Here's how the part is built. I have some questions about the finished solid (model axes, mm). Face numbers are marked on the shaded views. Round coordinates to 2 decimals unless told otherwise and drop trailing zeros. Loops run counter-clockwise (first coordinate to the right, second up) from the corner with the lowest first, then second, coordinate; pieces in that order, holes last. Notation, with made-up numbers: M 38.5,72.25 L 94.5,72.25 A15 ccw 94.5,77.25 Z; hole C 83.25,83.25 d7. An arc over 180 degrees is marked long. Use a Markdown table: item, result.
from build123d import *

# Parameters (mm, degrees)
SKETCH1_W                     = 262.636
SKETCH1_H                     = 3.175
BASE_FLANGE1_DEPTH            = 80.5688
CUT_EXTRUDE1_DEPTH            = 155.096817886
EDGE_FLANGE2_DEPTH            = 148.4376
EDGE_FLANGE3_DEPTH            = 249.936
EDGE_FLANGE4_DEPTH            = 148.4376
EDGE_FLANGE5_DEPTH            = 249.936
CSK_FOR_M5_SFHCS1_D           = 5.3
CSK_FOR_M5_SFHCS1_CSINK_D     = 11.2
CSK_FOR_M5_SFHCS1_CSINK_ANGLE = 90
CUT_EXTRUDE3_REACH            = 165.583
SKETCH18_W                    = 102.743
SKETCH18_H                    = 52.92295
FILLET2_R                     = 9.525
FILLET3_R                     = 6.35
FILLET4_R                     = 3.175


# Sheet-metal steps are written as plain solids
with BuildPart() as part:
    # Sketch1 → Base-Flange1 (new, symmetric)
    with BuildSketch(Plane.XY):
        with Locations((0, -1.5875)):
            Rectangle(SKETCH1_W, SKETCH1_H)
    extrude(amount=BASE_FLANGE1_DEPTH, both=True)

    # Sketch2 → Cut-Extrude1 (cut, through all)
    with BuildSketch(Plane(origin=(0, 0, 0), x_dir=(-1, 0, 0), z_dir=(0, 1, 0))):
        Polygon((131.318, -80.5688), (131.318, -74.2188), (124.968, -80.5688), align=None)
        Polygon((131.318, 74.2188), (124.968, 80.5688), (131.318, 80.5688), align=None)
        Polygon((-131.318, 80.5688), (-124.968, 80.5688), (-131.318, 74.2188), align=None)
        Polygon((-124.968, -80.5688), (-131.318, -80.5688), (-131.318, -74.2188), align=None)
    extrude(amount=-CUT_EXTRUDE1_DEPTH, mode=Mode.SUBTRACT)

    # Edge-Flange2 section (across the edge) → Edge-Flange2 (add)
    with BuildSketch(Plane(origin=(134.493, 0, 74.2188), x_dir=(-1, 0, 0), z_dir=(0, 0, -1))):
        with BuildLine():
            Line((-3.175, 3.175), (-3.175, 15.875))
            Line((-3.175, 15.875), (0, 15.875))
            Line((0, 15.875), (0, 3.175))
            ThreePointArc((0, 3.175), (0.92993597, 0.92993597), (3.175, 0))
            Line((3.175, 0), (3.175, -3.175))
            ThreePointArc((3.175, -3.175), (-1.315128061, -1.315128061), (-3.175, 3.175))
        make_face()
    extrude(amount=EDGE_FLANGE2_DEPTH)

    # Edge-Flange3 section (across the edge) → Edge-Flange3 (add)
    with BuildSketch(Plane(origin=(-124.968, 0, 83.7438), x_dir=(0, 0, -1), z_dir=(1, 0, 0))):
        with BuildLine():
            Line((-3.175, 3.175), (-3.175, 15.875))
            Line((-3.175, 15.875), (0, 15.875))
            Line((0, 15.875), (0, 3.175))
            ThreePointArc((0, 3.175), (0.92993597, 0.92993597), (3.175, 0))
            Line((3.175, 0), (3.175, -3.175))
            ThreePointArc((3.175, -3.175), (-1.315128061, -1.315128061), (-3.175, 3.175))
        make_face()
    extrude(amount=EDGE_FLANGE3_DEPTH)

    # Edge-Flange4 section (across the edge) → Edge-Flange4 (add)
    with BuildSketch(Plane(origin=(-134.493, 0, -74.2188), x_dir=(1, 0, 0), z_dir=(0, 0, 1))):
        with BuildLine():
            Line((-3.175, 3.175), (-3.175, 15.875))
            Line((-3.175, 15.875), (0, 15.875))
            Line((0, 15.875), (0, 3.175))
            ThreePointArc((0, 3.175), (0.92993597, 0.92993597), (3.175, 0))
            Line((3.175, 0), (3.175, -3.175))
            ThreePointArc((3.175, -3.175), (-1.315128061, -1.315128061), (-3.175, 3.175))
        make_face()
    extrude(amount=EDGE_FLANGE4_DEPTH)

    # Edge-Flange5 section (across the edge) → Edge-Flange5 (add)
    with BuildSketch(Plane(origin=(124.968, 0, -83.7438), x_dir=(0, 0, 1), z_dir=(-1, 0, 0))):
        with BuildLine():
            Line((-3.175, 3.175), (-3.175, 15.875))
            Line((-3.175, 15.875), (0, 15.875))
            Line((0, 15.875), (0, 3.175))
            ThreePointArc((0, 3.175), (0.92993597, 0.92993597), (3.175, 0))
            Line((3.175, 0), (3.175, -3.175))
            ThreePointArc((3.175, -3.175), (-1.315128061, -1.315128061), (-3.175, 3.175))
        make_face()
    extrude(amount=EDGE_FLANGE5_DEPTH)

    # CSK for M5 SFHCS1 (through all)
    with Locations(Plane.XZ.offset(3.175)):
        with Locations((-35, -15.75415), (35, -15.75415), (35, 2.24585), (-35, 2.24585)):
            CounterSinkHole(CSK_FOR_M5_SFHCS1_D / 2, CSK_FOR_M5_SFHCS1_CSINK_D / 2, counter_sink_angle=CSK_FOR_M5_SFHCS1_CSINK_ANGLE)

    # Sketch18 → Cut-Extrude3 (cut, up to next)
    with BuildSketch(Plane(origin=(0, 0, 0), x_dir=(1, 0, 0), z_dir=(0, 1, 0)), mode=Mode.PRIVATE) as cut_extrude3_sk1:
        with Locations((-60.8965, -41.407325)):
            Rectangle(SKETCH18_W, SKETCH18_H)
    cut_extrude3_tool1 = extrude(cut_extrude3_sk1.sketch, amount=-CUT_EXTRUDE3_REACH, mode=Mode.PRIVATE) & part.part
    # Sketch18 → Cut-Extrude3 (cut, up to next)
    with BuildSketch(Plane(origin=(0, 0, 0), x_dir=(1, 0, 0), z_dir=(0, 1, 0)), mode=Mode.PRIVATE) as cut_extrude3_sk2:
        with Locations((60.8965, -41.407325)):
            Rectangle(SKETCH18_W, SKETCH18_H)
    cut_extrude3_tool2 = extrude(cut_extrude3_sk2.sketch, amount=-CUT_EXTRUDE3_REACH, mode=Mode.PRIVATE) & part.part
    # Sketch18 → Cut-Extrude3 (cut, up to next)
    with BuildSketch(Plane(origin=(0, 0, 0), x_dir=(1, 0, 0), z_dir=(0, 1, 0)), mode=Mode.PRIVATE) as cut_extrude3_sk3:
        Polygon((-93.218, 28.45415), (-93.218, 10.45415), (-112.268, 10.45415), (-112.268, 65.62295), (-9.525, 65.62295), (-9.525, 28.45415), align=None)
    cut_extrude3_tool3 = extrude(cut_extrude3_sk3.sketch, amount=-CUT_EXTRUDE3_REACH, mode=Mode.PRIVATE) & part.part
    # Sketch18 → Cut-Extrude3 (cut, up to next)
    with BuildSketch(Plane(origin=(0, 0, 0), x_dir=(1, 0, 0), z_dir=(0, 1, 0)), mode=Mode.PRIVATE) as cut_extrude3_sk4:
        Polygon((9.525, 65.62295), (112.268, 65.62295), (112.268, 10.45415), (93.218, 10.45415), (93.218, 28.45415), (9.525, 28.45415), align=None)
    cut_extrude3_tool4 = extrude(cut_extrude3_sk4.sketch, amount=-CUT_EXTRUDE3_REACH, mode=Mode.PRIVATE) & part.part
    add(cut_extrude3_tool1.solids().sort_by_distance((-60.8965, 0, 41.407325))[0], mode=Mode.SUBTRACT)
    add(cut_extrude3_tool2.solids().sort_by_distance((60.8965, 0, 41.407325))[0], mode=Mode.SUBTRACT)
    add(cut_extrude3_tool3.solids().sort_by_distance((-64.344381, 0, -44.765774))[0], mode=Mode.SUBTRACT)
    add(cut_extrude3_tool4.solids().sort_by_distance((64.344381, 0, -44.765774))[0], mode=Mode.SUBTRACT)

    # Fillet2
    fillet2_edges = [part.edges().sort_by_distance(p)[0] for p in [
        (112.268, -1.5875, 14.94585),
        (112.268, -1.5875, 67.8688),
        (9.525, -1.5875, 67.8688),
        (9.525, -1.5875, 14.94585),
        (-112.268, -1.5875, -65.62295),
        (-9.525, -1.5875, -65.62295),
        (-9.525, -1.5875, -28.45415),
        (-93.218, -1.5875, -28.45415),
        (9.525, -1.5875, -28.45415),
        (9.525, -1.5875, -65.62295),
        (112.268, -1.5875, -65.62295),
        (93.218, -1.5875, -28.45415),
        (-9.525, -1.5875, 14.94585),
        (-9.525, -1.5875, 67.8688),
        (-112.268, -1.5875, 67.8688),
        (-112.268, -1.5875, 14.94585),
    ]]
    fillet(fillet2_edges, radius=FILLET2_R)

    # Fillet3
    fillet3_edges = [part.edges().sort_by_distance(p)[0] for p in [
        (-112.268, -1.5875, -10.45415),
        (-93.218, -1.5875, -10.45415),
        (112.268, -1.5875, -10.45415),
        (93.218, -1.5875, -10.45415),
    ]]
    fillet(fillet3_edges, radius=FILLET3_R)

    # Fillet4
    fillet4_edges = [part.edges().sort_by_distance(p)[0] for p in [
        (-136.0805, 15.875, -74.2188),
        (-136.0805, 15.875, 74.2188),
        (124.968, 15.875, -85.3313),
        (-124.968, 15.875, -85.3313),
        (136.0805, 15.875, 74.2188),
        (136.0805, 15.875, -74.2188),
        (-124.968, 15.875, 85.3313),
        (124.968, 15.875, 85.3313),
    ]]
    fillet(fillet4_edges, radius=FILLET4_R)


solid = part.part
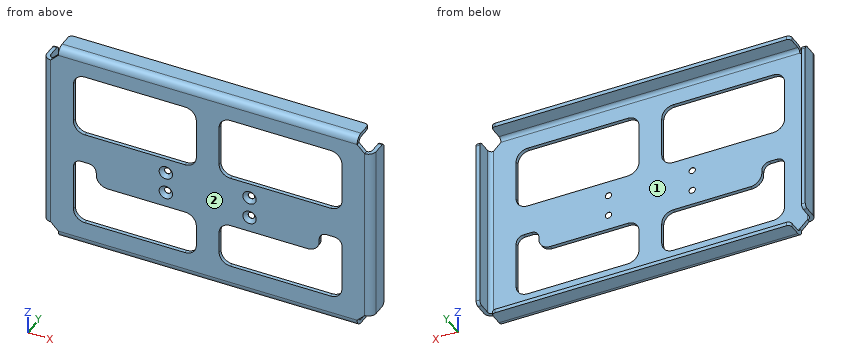
1. Imagine slicing it at B-B, the plane z = -43. Write out the boundary of the cut face in (x, y) (3 decimals), then the cut area to 3 significant figures.
Answer sheet:
| item | result |
|---|---|
| outline | M -137.668,3.175 A6.35 ccw -131.318,-3.175 L -112.268,-3.175 L -112.268,0 L -131.318,0 A3.175 cw -134.493,3.175 L -134.493,15.875 L -137.668,15.875 Z; M -9.525,-3.175 L 9.525,-3.175 L 9.525,0 L -9.525,0 Z; M 112.268,-3.175 L 131.318,-3.175 A6.35 ccw 137.668,3.175 L 137.668,15.875 L 134.493,15.875 L 134.493,3.175 A3.175 cw 131.318,0 L 112.268,0 Z |
| area | 310 mm2 |
2. We'd pull the mould along X, two halves only. Please class the marked faces 1 and 2: +X half, -X half, draft (parallel to the pull), parting line (faces both ways), or undercut.
Answer sheet:
| item | result |
|---|---|
| face 1 | undercut |
| face 2 | draft |
3. Imagine slicing it at A-A, the plane x = -24. Write out the boundary of the cut face in (y, z) (3 decimals), then the cut area to 3 significant figures.
Answer sheet:
| item | result |
|---|---|
| outline | M -3.175,-80.569 A6.35 ccw 3.175,-86.919 L 15.875,-86.919 L 15.875,-83.744 L 3.175,-83.744 A3.175 cw 0,-80.569 L 0,-65.623 L -3.175,-65.623 Z; M -3.175,-28.454 L 0,-28.454 L 0,14.946 L -3.175,14.946 Z; M -3.175,67.869 L 0,67.869 L 0,80.569 A3.175 cw 3.175,83.744 L 15.875,83.744 L 15.875,86.919 L 3.175,86.919 A6.35 ccw -3.175,80.569 Z |
| area | 354 mm2 |
4. I need wall thicknesses on probe 1 along X at (y, z) = (4.5, 61.5); probe 2 along Z at (x, y) = (29, 12.25); probe 3 along Z at (x, y) = (35, -0.05). Which ranges of each line are inside material? Lowest first, please. Write a range as from..to.
Answer sheet:
| item | result |
|---|---|
| probe 1 | -137.67..-134.49, 134.49..137.67 |
| probe 2 | -86.92..-83.74, 83.74..86.92 |
| probe 3 | -86.04..-65.62, -28.45..-18.4, -13.1..-0.4, 4.9..14.95, 67.87..86.04 |
5. Imagine slicing it at D-D, the plane x = 35. State how many separate pieces and enclosed holes the cut face has, then the cut area to 3 significant figures.
Answer sheet:
| item | result |
|---|---|
| separate pieces | 5 |
| enclosed holes | 0 |
| area | 303 mm2 |
6. Imagine slicing it at C-C, the plane y = 8.5. Write out the boundary of the cut face in (x, z), then the cut area to 3 significant figures.
Answer sheet:
| item | result |
|---|---|
| outline | M -137.67,-74.22 L -134.49,-74.22 L -134.49,74.22 L -137.67,74.22 Z; M -124.97,-86.92 L 124.97,-86.92 L 124.97,-83.74 L -124.97,-83.74 Z; M -124.97,83.74 L 124.97,83.74 L 124.97,86.92 L -124.97,86.92 Z; M 134.49,-74.22 L 137.67,-74.22 L 137.67,74.22 L 134.49,74.22 Z |
| area | 2,530 mm2 |
7. For pin 1 Ø5 at (x, z) = (-61.5, 67.5) entering from +Y; pin 2 Ø2.5 at (y, z) = (-2.5, -47.5) entering from -X; pin 3 Ø3.5 at (x, y) = (60, -1.5) entering from -Z (3 decimals), each with a flat end and sliding along its axis, tell me the tip position at first contact or that it passes through.
Answer sheet:
| item | result |
|---|---|
| pin 1 | y = 0 |
| pin 2 | x = -135.87 |
| pin 3 | z = -86.205 |
